```python
from build123d import *

# Parameters (mm, degrees)
F0_R     = 1.2813159657
F1_DEPTH = 7.5
F2_DEPTH = 5.25


# Not quite as in the source:
# - ends of sketch curves that miss each other by under 0.0002 mm in the source are joined


with BuildPart() as f1:
    # F0 (on Front) → F1 (new body, symmetric)
    with BuildSketch(Plane.XZ):
        with BuildLine():
            ThreePointArc((7.8928847665, 2.2551549829), (-0.5468394213, 4.4913902739), (-9.2777672646, 4.515713911))
            Line((-9.2777672646, 4.515713911), (-9.27776646, -6.4638420574))
            ThreePointArc((-9.27776646, -6.4638420574), (-8.7082936227, -7.7372240383), (-7.3795216285, -8.1616848044))
            ThreePointArc((-7.3795216285, -8.1616848044), (-2.2192897787, -8.212150504), (2.7781677389, -9.4989699664))
            ThreePointArc((2.7781677389, -9.4989699664), (4.1715212346, -9.432884372), (5.0511658084, -8.3502824825))
            Line((5.0511658084, -8.3502824825), (7.8928847665, 2.2551549829))
        make_face()
        with Locations((-5.0067132411, -3.7583980654)):
            Circle(F0_R, mode=Mode.SUBTRACT)
        with Locations((1.6258659514, -4.6315961033)):
            Circle(F0_R, mode=Mode.SUBTRACT)
        with BuildLine():
            Line((8.8106123745, 5.6801667894), (-9.27776646, 8.0615492201))
            Line((-9.27776646, 8.0615492201), (-9.27776646, 4.515713911))
            ThreePointArc((-9.27776646, 4.515713911), (-0.5468394213, 4.4913902739), (7.8928847665, 2.2551549829))
            Line((7.8928847665, 2.2551549829), (8.8106123745, 5.6801667894))
        make_face()
    extrude(amount=F1_DEPTH, both=True)

    # F0 (on Front) → F2 (cut, symmetric)
    with BuildSketch(Plane.XZ):
        with BuildLine():
            ThreePointArc((7.8928847665, 2.2551549829), (-0.5468394213, 4.4913902739), (-9.2777672646, 4.515713911))
            Line((-9.2777672646, 4.515713911), (-9.27776646, -6.4638420574))
            ThreePointArc((-9.27776646, -6.4638420574), (-8.7082936227, -7.7372240383), (-7.3795216285, -8.1616848044))
            ThreePointArc((-7.3795216285, -8.1616848044), (-2.2192897787, -8.212150504), (2.7781677389, -9.4989699664))
            ThreePointArc((2.7781677389, -9.4989699664), (4.1715212346, -9.432884372), (5.0511658084, -8.3502824825))
            Line((5.0511658084, -8.3502824825), (7.8928847665, 2.2551549829))
        make_face()
        with Locations((-5.0067132411, -3.7583980654)):
            Circle(F0_R, mode=Mode.SUBTRACT)
        with Locations((1.6258659514, -4.6315961033)):
            Circle(F0_R, mode=Mode.SUBTRACT)
        with Locations((-5.0067132411, -3.7583980654)):
            Circle(F0_R)
        with Locations((1.6258659514, -4.6315961033)):
            Circle(F0_R)
    extrude(amount=F2_DEPTH, both=True, mode=Mode.SUBTRACT)


solid = f1.part
```
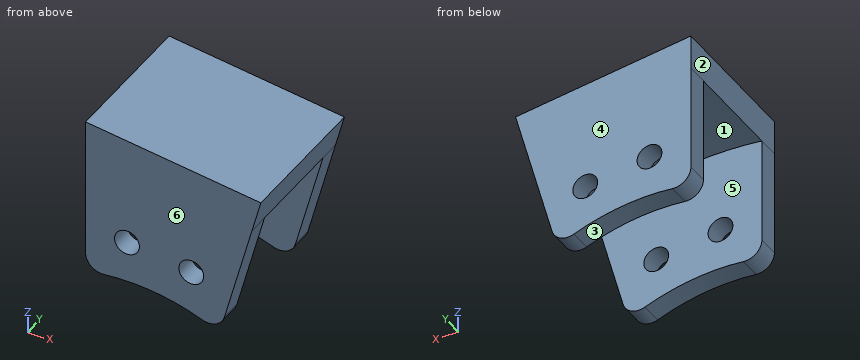
Verification items for the finished model (mm, model axes). Face numbers are marked on the shaded views. A direction names the side the tool comes from. Give positions to 0.01 mm unless a question says otherwise; leave off trailing zeros. Order: outer loops, then holes, each group sorted by start corner. A loop starts at its lowest first (then second) coordinate and runs counter-clockwise, first axis right, second up. Notation, with made-up numbers: M 70.25,84 L 102.25,84 A17 ccw 102.25,102 Z; hole C 33,18 d10. An arc over 180 degrees is marked long. Return JSON: item names as keys, results as strings. Group by question number.
1) Section check C-C on z = 3. Record the cut outline in (x, y), and give its area (3 significant figures).
2) Access from +Z, -Z, +X, -X, +Y, -Y to the whole of each face (thin tool, end or side, straight path). Record for the marked faces 1 and 2.
3) Mould release check, pull along Y, two halves, no side actions. Record for the marked faces 3, 4, 5 and 6: pulls with the +Y half, pulls with the -Y half, needs draft (parallel to the pull), parting line crosses it, or undercut.
4) Section check B-B on x = -7.75. Record the cut outline in (y, z).
5) Section check D-D on y = -2. Record the cut outline in (x, z).
6) Section check A-A on z = -0.5. Record the cut outline in (x, y), and give its area (3 significant figures).
7) Scan lines: line 1 (Y direction, x = -5.5, z = 3); line 2 (Z direction, x = -5, y = 2.5); line 3 (Z direction, x = 1.75, y = 4.25). Record each from-to range of solid material in increasing order.
8) Go/stop test with flat-tipped pins: pin 1 Ø1.5 at (x, z) = (-5.01, -3.76) entering from -Y; pin 2 Ø1.5 at (x, y) = (-7.5, 2.5) entering from -Z; pin 3 Ø3 at (y, z) = (4.5, -1) entering from +X. Record where each tip stops, or that it passes through.
Answer block:
{
 "1": {"outline": "M -9.28,-7.5 L 8.09,-7.5 L 8.09,7.5 L -9.28,7.5 L -9.28,5.25 L 5.89,5.25 L 5.89,-5.25 L -9.28,-5.25 Z", "area": "101 mm^2"},
 "2": {"face 1": "-Z", "face 2": "+Z, -Z, -X, +Y, -Y"},
 "3": {"face 3": "needs draft", "face 4": "pulls with the +Y half", "face 5": "undercut", "face 6": "pulls with the -Y half"},
 "4": {"outline": "M -7.5,-8.16 L -5.25,-8.16 L -5.25,4.67 L 5.25,4.67 L 5.25,-8.16 L 7.5,-8.16 L 7.5,7.86 L -7.5,7.86 Z"},
 "5": {"outline": "M -9.28,4.52 A34.17 cw 7.89,2.26 L 8.81,5.68 L -9.28,8.06 Z"},
 "6": {"outline": "M -9.28,-7.5 L 7.15,-7.5 L 7.15,-5.25 L -9.28,-5.25 Z; M -9.28,5.25 L 7.15,5.25 L 7.15,7.5 L -9.28,7.5 Z", "area": "73.9 mm^2"},
 "7": {"line 1": "y = -7.5 to -5.25, 5.25 to 7.5", "line 2": "z = 4.78 to 7.5", "line 3": "z = 4.11 to 6.61"},
 "8": {"pin 1": "passes through", "pin 2": "stops at z = 4.63", "pin 3": "stops at x = 7.37"}
}
